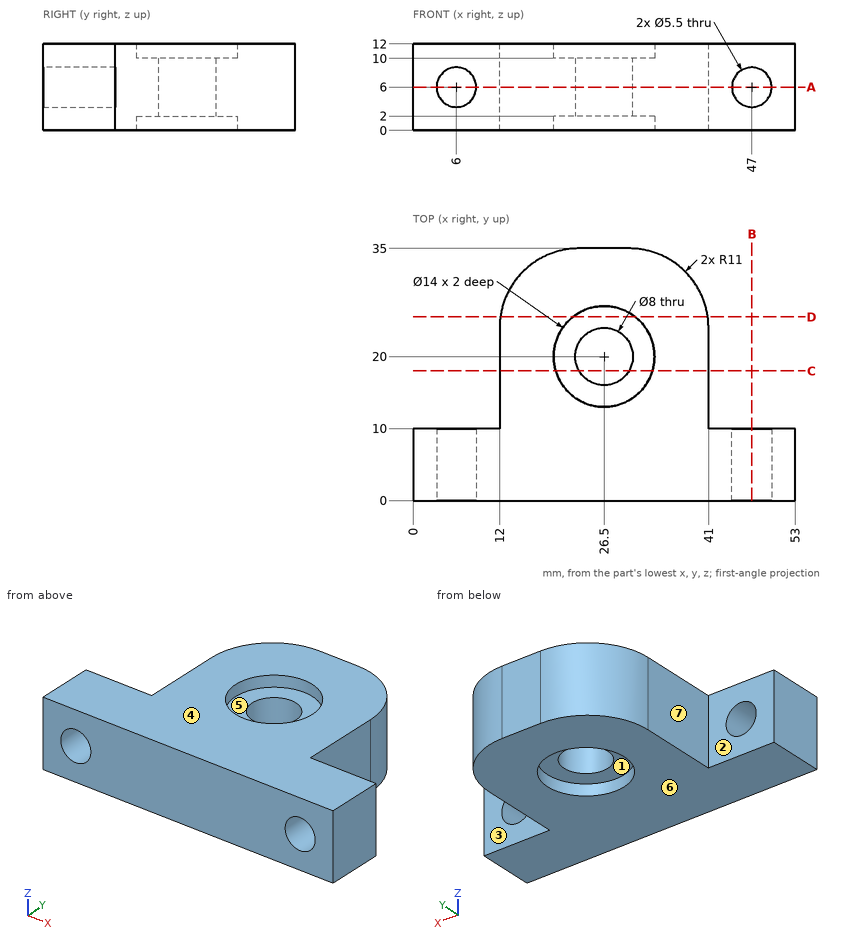
Can you work these out from the drawing? Everything is in mm from the part's minimum corner. A direction names the side the tool comes from. Round coordinates to 2 decimals unless told otherwise and drop trailing zeros. Loops run counter-clockwise (first coordinate to the right, second up) from the corner with the lowest first, then second, coordinate; pieces in that order, holes last. Notation, with made-up numbers: (67, 50.25) - (117, 50.25) arc R23 ccw to (117, 66.25) - close; hole circle Ø11 at (81, -7.75). An arc over 180 degrees is marked (long way). One line per question, with ' | ' between items. Start each with the question number.
Q1. I want a section at D-D (y = 25.5). Write out the boundary of the cut face in (x, z), then the cut area to 3 significant figures.
Q2. Please list where these lines run through material, in increasing order: line 1 (X direction, y = 6.5, z = 6); line 2 (Z direction, x = 47, y = 4); line 3 (X direction, y = 20, z = 9.75). Write a range as [from, to].
Q3. I want a section at C-C (y = 18). Write out the boundary of the cut face in (x, z).
Q4. I want a section at B-B (x = 47). Write out the boundary of the cut face in (y, z), then the cut area to 3 significant figures.
Q5. I want a section at A-A (z = 6). Write out the boundary of the cut face in (x, y), then the cut area to 3 significant figures.
Q6. We'd pull the mould along X, two halves only. Please class the marked faces 5, 6 and 7: +X half, -X half, draft (parallel to the pull), parting line (faces both ways), or undercut.
Q7. For the marked faces 1, 2, 3 and 4, which set-ups out of +Z, -Z, +X, -X, +Y, -Y let a thin tool reach every point of the face, with its end or its side?
Q8. Will these pins go through, and if not, where does the flat tip stop? pin 1 (6 mm diameter, centred on x = 20, y = 15.5, fed in from -Z); pin 2 (11 mm diameter, centred on x = 26.5, y = 20, fed in from +Z); pin 3 (3 mm diameter, centred on x = 16.5, z = 9, fed in from +Y); pin 4 (3.5 mm diameter, centred on x = 46, z = 5, fed in from +Y).
Response values:
1) outline: (12.1, 0) - (22.17, 0) - (22.17, 2) - (30.83, 2) - (30.83, 0) - (40.9, 0) - (40.9, 12) - (30.83, 12) - (30.83, 10) - (22.17, 10) - (22.17, 12) - (12.1, 12) - close | area: 311 mm²
2) line 1: x = [0, 3.25], [8.75, 44.25], [49.75, 53] | line 2: z = [0, 3.25], [8.75, 12] | line 3: x = [12, 22.5], [30.5, 41]
3) outline: (12, 0) - (19.79, 0) - (19.79, 2) - (23.04, 2) - (23.04, 10) - (19.79, 10) - (19.79, 12) - (12, 12) - close; (29.96, 2) - (33.21, 2) - (33.21, 0) - (41, 0) - (41, 12) - (33.21, 12) - (33.21, 10) - (29.96, 10) - close
4) outline: (0, 0) - (10, 0) - (10, 3.25) - (0, 3.25) - close; (0, 8.75) - (10, 8.75) - (10, 12) - (0, 12) - close | area: 65.0 mm²
5) outline: (0, 0) - (3.25, 0) - (3.25, 10) - (0, 10) - close; (8.75, 0) - (44.25, 0) - (44.25, 10) - (41, 10) - (41, 24) arc R11 ccw to (30, 35) - (23, 35) arc R11 ccw to (12, 24) - (12, 10) - (8.75, 10) - close; (49.75, 0) - (53, 0) - (53, 10) - (49.75, 10) - close; hole circle Ø8 at (26.5, 20) | area: 1,040 mm²
6) face 5: undercut | face 6: draft | face 7: -X half
7) face 1: -Z | face 2: +Z, -Z, -X, +Y | face 3: +Z, -Z, +X, +Y | face 4: +Z, +X, -X, +Y, -Y
8) pin 1: stops at z = 0 | pin 2: stops at z = 10 | pin 3: stops at y = 33.8 | pin 4: stops at y = 10
